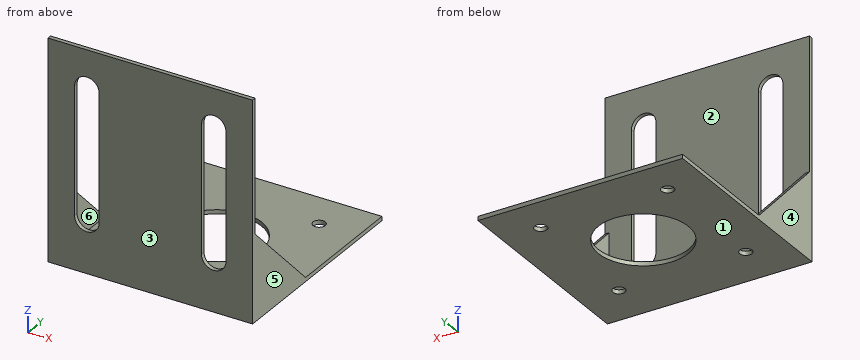
```python
from build123d import *

# Parameters (mm, degrees)
SKETCH_1_W          = 50
SKETCH_1_H          = 53.5
EXTRUDE_1_DEPTH     = 1
SKETCH_2_W          = 50
SKETCH_2_H          = 51.3
SKETCH_2_R          = 1.5
EXTRUDE_2_DEPTH     = 1
EXTRUDE_3_DEPTH     = 1
EXTRUDE_4_DEPTH     = 1
SKETCH_7_R          = 11
CUT_EXTRUDE_1_DEPTH = 78.543149278


with BuildPart() as part:
    # 草图1 → 凸台-拉伸1 (new body)
    with BuildSketch(Plane(origin=(0, 0, 0), x_dir=(1, 0, 0), z_dir=(0, 1, 0))):
        Rectangle(SKETCH_1_W, SKETCH_1_H)
        with BuildLine():
            Line((-18.5, 13.75), (-18.5, -17.25))
            ThreePointArc((-18.5, -17.25), (-15.5, -20.25), (-12.5, -17.25))
            Line((-12.5, -17.25), (-12.5, 13.75))
            ThreePointArc((-12.5, 13.75), (-15.5, 16.75), (-18.5, 13.75))
        make_face(mode=Mode.SUBTRACT)
        with BuildLine():
            Line((12.5, 13.75), (12.5, -17.25))
            ThreePointArc((12.5, -17.25), (15.5, -20.25), (18.5, -17.25))
            Line((18.5, -17.25), (18.5, 13.75))
            ThreePointArc((18.5, 13.75), (15.5, 16.75), (12.5, 13.75))
        make_face(mode=Mode.SUBTRACT)
    extrude(amount=EXTRUDE_1_DEPTH)

    # 草图2 → 凸台-拉伸2 (add)
    with BuildSketch(Plane.XY.offset(-26.75)):
        with Locations((0, 25.65)):
            Rectangle(SKETCH_2_W, SKETCH_2_H)
        with Locations((-15.5, 41.8)):
            Circle(SKETCH_2_R, mode=Mode.SUBTRACT)
        with Locations((15.5, 41.8)):
            Circle(SKETCH_2_R, mode=Mode.SUBTRACT)
        with Locations((-15.5, 10.8)):
            Circle(SKETCH_2_R, mode=Mode.SUBTRACT)
        with Locations((15.5, 10.8)):
            Circle(SKETCH_2_R, mode=Mode.SUBTRACT)
    extrude(amount=EXTRUDE_2_DEPTH)

    # 草图4 → 凸台-拉伸3 (add)
    with BuildSketch(Plane(origin=(-25, 0, 0), x_dir=(0, 0, -1), z_dir=(1, 0, 0))):
        Polygon((25.75, 21), (5.75, 1), (25.75, 1), align=None)
    extrude(amount=EXTRUDE_3_DEPTH)

    # 草图6 → 凸台-拉伸4 (add)
    with BuildSketch(Plane.ZY.offset(-25)):
        Polygon((-25.75, 21), (-5.75, 1), (-25.75, 1), align=None)
    extrude(amount=EXTRUDE_4_DEPTH)

    # 草图7 → 切除-拉伸1 (cut, through all)
    with BuildSketch(Plane.XY.offset(-25.75)):
        with Locations((0, 26.3)):
            Circle(SKETCH_7_R)
    extrude(amount=-CUT_EXTRUDE_1_DEPTH, mode=Mode.SUBTRACT)


solid = part.part
```
The model under review builds one solid part; all positions refer to its coordinate system, in mm. Face numbers are marked on the shaded views. A direction names the side the tool comes from. Give positions to 0.01 mm unless a question says otherwise; leave off trailing zeros. Write each loop counter-clockwise with the first axis right and the second up, starting at its lowest first coordinate (ties: lowest second). Pieces come first, ordered by that corner, then holes. Notation, with made-up numbers: (77.25, 42) -> (107.25, 42) arc R12 ccw to (107.25, 55) -> close; hole circle Ø1 at (17.5, 35.5). An arc over 180 degrees is marked (long way). Answer in a Markdown table with one row per item.
1) Mouldability with a two-part tool opening along X and no side actions: class the marked faces 3, 4, 5 and 6 as +X half, -X half, draft (parallel to the pull), parting line (faces both ways), or undercut.
Worked answers:
| item | result |
|---|---|
| face 3 | draft |
| face 4 | -X half |
| face 5 | +X half |
| face 6 | undercut |
2) For L1, parallel to Y at x = 0, z = -26.1; L2, parallel to Y at x = 15.5, z = -26.1; L3, parallel to Y at x = -15, z = -26, list the stretches that pass through material, from the lowest coordinate up. Write a range as [from, to].
Worked answers:
| item | result |
|---|---|
| L1 | [0, 15.3], [37.3, 51.3] |
| L2 | [0, 9.3], [12.3, 40.3], [43.3, 51.3] |
| L3 | [0, 9.39], [12.21, 40.39], [43.21, 51.3] |
3) Tool access review of the marked faces 1 and 2: name each direction out of +Z, -Z, +X, -X, +Y, -Y from which nothing blocks a thin tool from reaching the whole face with its end or side.
Worked answers:
| item | result |
|---|---|
| face 1 | -Z, +X, -X, +Y, -Y |
| face 2 | +Z, +Y |
4) Clearance check with flat-ended pins moving along their axes: P1, Ø1, axis at x = 13, y = 36.5, coming from the +Z side; P2, Ø10, axis at x = 10.5, z = 16.5, coming from the -Y side; P3, Ø15, axis at x = 1, z = 10, coming from the +Y side. State where each tip first meets the part, or that it passes through.
Worked answers:
| item | result |
|---|---|
| P1 | z = -25.75 |
| P2 | y = 0 |
| P3 | y = 1 |
5) Add section D-D on x = 0. State the section outline as (y, z) points.
Worked answers:
| item | result |
|---|---|
| outline | (0, -26.75) -> (15.3, -26.75) -> (15.3, -25.75) -> (1, -25.75) -> (1, 26.75) -> (0, 26.75) -> close; (37.3, -26.75) -> (51.3, -26.75) -> (51.3, -25.75) -> (37.3, -25.75) -> close |
6) Add section A-A on z = -12.5. State the section outline as (x, y) points.
Worked answers:
| item | result |
|---|---|
| outline | (-25, 0) -> (-18.5, 0) -> (-18.5, 1) -> (-24, 1) -> (-24, 7.75) -> (-25, 7.75) -> close; (-12.5, 0) -> (12.5, 0) -> (12.5, 1) -> (-12.5, 1) -> close; (18.5, 0) -> (25, 0) -> (25, 7.75) -> (24, 7.75) -> (24, 1) -> (18.5, 1) -> close |
7) Add section B-B on x = -15.5. State the section outline as (y, z) points, plus the area to 3 significant figures.
Worked answers:
| item | result |
|---|---|
| outline | (0, -26.75) -> (9.3, -26.75) -> (9.3, -25.75) -> (1, -25.75) -> (1, -16.75) -> (0, -16.75) -> close; (0, 20.25) -> (1, 20.25) -> (1, 26.75) -> (0, 26.75) -> close; (12.3, -26.75) -> (40.3, -26.75) -> (40.3, -25.75) -> (12.3, -25.75) -> close; (43.3, -26.75) -> (51.3, -26.75) -> (51.3, -25.75) -> (43.3, -25.75) -> close |
| area | 60.8 mm² |
8) Add section C-C on y = 10.8. State the section outline as (x, z) points.
Worked answers:
| item | result |
|---|---|
| outline | (-25, -26.75) -> (-17, -26.75) -> (-17, -25.75) -> (-24, -25.75) -> (-24, -15.55) -> (-25, -15.55) -> close; (-14, -26.75) -> (14, -26.75) -> (14, -25.75) -> (-14, -25.75) -> close; (17, -26.75) -> (25, -26.75) -> (25, -15.55) -> (24, -15.55) -> (24, -25.75) -> (17, -25.75) -> close |
